The figure shows three views and two pictorial views of one solid part (mm, origin at its lowest corner). Answer the questions. A direction names the side the tool comes from. Coordinates: 2 decimals unless noted, no trailing zeros. Order: outer loops, then holes, each group sorted by start corner. A loop starts at its lowest first (then second) coordinate and runs counter-clockwise, first axis right, second up. Notation, with made-up numbers: (71, 71.25) - (110, 71.25) arc R14 cw to (110, 84.25) - close; hole circle Ø5 at (1.25, -3). An arc over 180 degrees is marked (long way). Use one line per item in the form item = value. Start each with the question number.
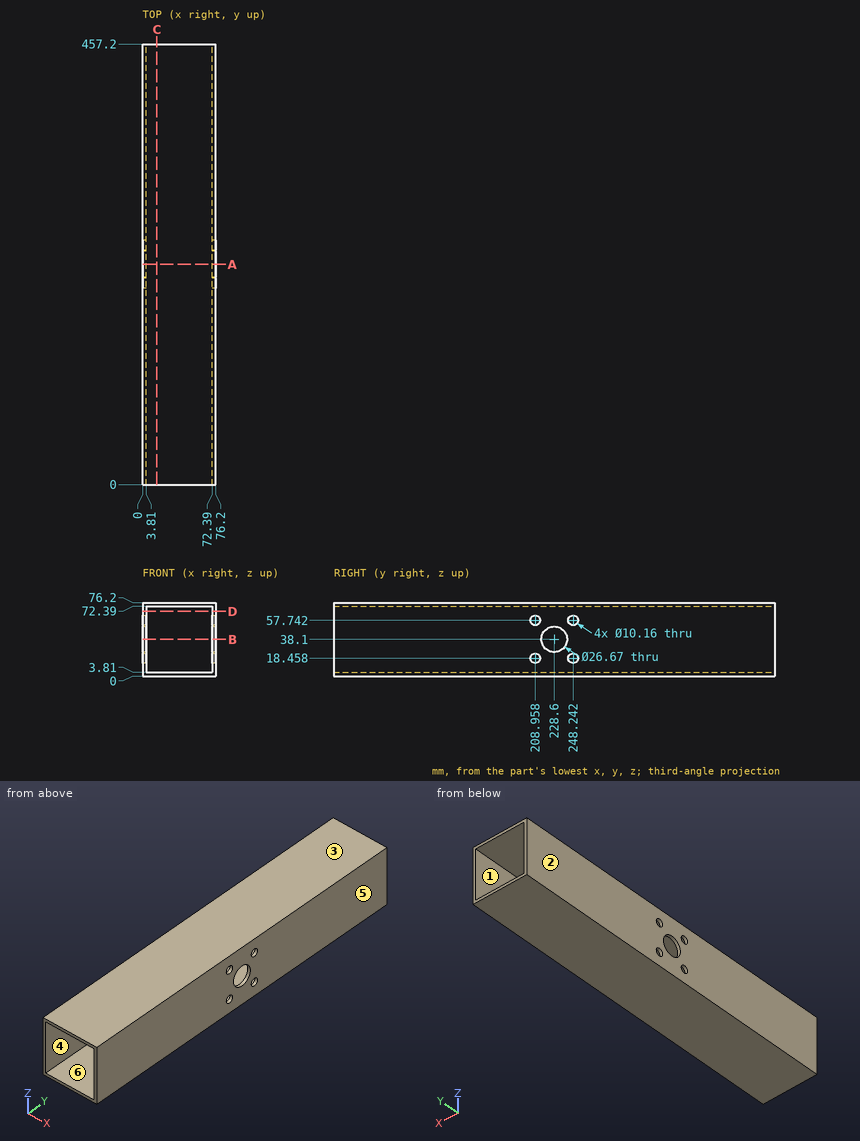
Q1. A cutting plane is placed at D-D (z = 67). Give the vertices of the cut face in (x, y).
Q2. Which of the six approach directions +Z, -Z, +X, -X, +Y, -Y give full straight-line access (tool end or side, diameter ignored) to the marked faces 1 and 2?
Q3. A cutting plane is placed at B-B (z = 38.1). Give the vertices of the cut face in (x, y) (1 decimal).
Q4. For a pull along Z with two mould halves and no side action, classify the marked faces 3, 4, 5 and 6 as +Z half, -Z half, draft (parallel to the pull), parting line (faces both ways), or undercut.
Q5. A cutting plane is placed at A-A (y = 228.6). Give the vertices of the cut face in (x, z) (1 decimal), then the cut area to 3 significant figures.
Q6. A cutting plane is placed at C-C (x = 15). Give the vertices of the cut face in (y, z).
Q7. Consider probe 1 along Z at (x, y) = (8, 248.5). Determine where the line is inside the solid, lowest interval first.
Q8. Given P1, Ø13, axis at y = 208.96, z = 57.74, coming from the +X side; P2, Ø9, axis at y = 208.96, z = 18.46, coming from the +X side, each flat-ended and moving along its own axis, determine where each tip first touches the part or whether it passes through.
Result sheet:
q1.outline = (0, 0) - (3.81, 0) - (3.81, 457.2) - (0, 457.2) - close; (72.39, 0) - (76.2, 0) - (76.2, 457.2) - (72.39, 457.2) - close
q2.face_1 = +Y, -Y
q2.face_2 = +Z, -Z, -X, +Y, -Y
q3.outline = (0, 0) - (3.8, 0) - (3.8, 215.3) - (0, 215.3) - close; (0, 241.9) - (3.8, 241.9) - (3.8, 457.2) - (0, 457.2) - close; (72.4, 0) - (76.2, 0) - (76.2, 215.3) - (72.4, 215.3) - close; (72.4, 241.9) - (76.2, 241.9) - (76.2, 457.2) - (72.4, 457.2) - close
q4.face_3 = +Z half
q4.face_4 = undercut
q4.face_5 = draft
q4.face_6 = undercut
q5.outline = (0, 0) - (76.2, 0) - (76.2, 24.8) - (72.4, 24.8) - (72.4, 3.8) - (3.8, 3.8) - (3.8, 24.8) - (0, 24.8) - close; (0, 51.4) - (3.8, 51.4) - (3.8, 72.4) - (72.4, 72.4) - (72.4, 51.4) - (76.2, 51.4) - (76.2, 76.2) - (0, 76.2) - close
q5.area = 900 mm^2
q6.outline = (0, 0) - (457.2, 0) - (457.2, 3.81) - (0, 3.81) - close; (0, 72.39) - (457.2, 72.39) - (457.2, 76.2) - (0, 76.2) - close
q7.probe_1 = 0 to 3.81, 72.39 to 76.2
q8.P1 = 76.2
q8.P2 = through
